Work out the finished part from the listing and answer in its coordinate system (mm). A direction names the side the tool comes from. Give positions to 0.01 mm unless a question says otherwise; leave off trailing zeros. Order: outer loops, then holes, each group sorted by start corner. A loop starts at its lowest first (then second) coordinate and runs counter-clockwise, first axis right, second up. Notation, with made-up numbers: (-4, 7.5) -> (43, 7.5) arc R28 ccw to (43, 36.5) -> close; hole circle Ø1 at (-23, 37). An arc over 180 degrees is marked (long way). Use a Markdown table: item, result. Add a question column.
```python
from build123d import *

# Parameters (mm, degrees)
F0_W     = 32.913417
F0_H     = 15.983271
F0_R     = 0.5
F0_R_2   = 1
F0_R_3   = 1.5
F0_R_4   = 2
F0_R_5   = 2.5
F1_DEPTH = 2
F2_R     = 0.5
F2_R_2   = 1
F2_R_3   = 1.5
F2_R_4   = 2
F2_R_5   = 2.5
F3_DEPTH = 2


with BuildPart() as f1:
    # F0 (on Top) → F1 (new body)
    with BuildSketch(Plane.XY):
        with Locations((16.456708, 7.991635)):
            Rectangle(F0_W, F0_H)
        with Locations((3.5, 3.5)):
            Circle(F0_R, mode=Mode.SUBTRACT)
        with Locations((7.972136, 4)):
            Circle(F0_R_2, mode=Mode.SUBTRACT)
        with Locations((13.449362, 4.5)):
            Circle(F0_R_3, mode=Mode.SUBTRACT)
        with Locations((19.930102, 5)):
            Circle(F0_R_4, mode=Mode.SUBTRACT)
        with Locations((27.413417, 5.5)):
            Circle(F0_R_5, mode=Mode.SUBTRACT)
        with Locations((5.5, 10.483271)):
            Circle(F0_R_5, mode=Mode.SUBTRACT)
        with Locations((12.983315, 10.983271)):
            Circle(F0_R_4, mode=Mode.SUBTRACT)
        with Locations((19.464055, 11.483271)):
            Circle(F0_R_3, mode=Mode.SUBTRACT)
        with Locations((24.941281, 11.983271)):
            Circle(F0_R_2, mode=Mode.SUBTRACT)
        with Locations((29.413417, 12.483271)):
            Circle(F0_R, mode=Mode.SUBTRACT)
        with Locations((5.5, 10.483271)):
            Circle(F0_R_5)
        with Locations((12.983315, 10.983271)):
            Circle(F0_R_4)
        with Locations((19.464055, 11.483271)):
            Circle(F0_R_3)
        with Locations((24.941281, 11.983271)):
            Circle(F0_R_2)
        with Locations((29.413417, 12.483271)):
            Circle(F0_R)
    extrude(amount=F1_DEPTH)

    # F2 (on face) → F3 (join)
    with BuildSketch(Plane.XY.offset(2)):
        with Locations((29.413417, 12.483271)):
            Circle(F2_R)
        with Locations((24.941281, 11.983271)):
            Circle(F2_R_2)
        with Locations((19.464055, 11.483271)):
            Circle(F2_R_3)
        with Locations((12.983315, 10.983271)):
            Circle(F2_R_4)
        with Locations((5.5, 10.483271)):
            Circle(F2_R_5)
    extrude(amount=F3_DEPTH)


solid = f1.part
```
1) Flat-ended cylindrical pins translate along their axes: pin 1 (5 mm diameter, centred on x = 28, y = 4, fed in from +Z); pin 2 (4.5 mm diameter, centred on x = 27.41, y = 5.5, fed in from +Z); pin 3 (1 mm diameter, centred on y = 12, z = 3.5, fed in from -X). Find the tip coordinate at first contact, or state that the pin passes through.
2) The part is cut by section B-B, the plane x = 8.5. Determine the outline of the cut face in (y, z), then the cut area to 3 significant figures.
3) The part is cut by section A-A, the plane y = 7.5. Determine the outline of the cut face in (x, z).
4) Which of the six approach directions +Z, -Z, +X, -X, +Y, -Y give full straight-line access (tool end or side, diameter ignored) to faces 5 (the cylindrical face through (17.966, 11.549, 2.986)), 6 (the cylindrical face through (14.835, 3.925, 0.986))?
5) Straight lines are drawn through the part: line 1 (Z direction, x = 29.5, y = 10.5); line 2 (Y direction, x = 28.5, z = 1.5); line 3 (Y direction, x = 19.5, z = 3.35). For each, find the intervals that lie inside material, in ascending order.
6) The part is cut by section C-C, the plane z = 1.1. Determine the outline of the cut face in (x, y).
7) The part is cut by section D-D, the plane y = 4.5. Determine the outline of the cut face in (x, z).
8) Determine the mould class of faces 1 (the flat face through (0, 8, 1)), 2 (the cylindrical face through (14.891, 11.584, 2.986)), 3 (the flat face through (32.913, 8, 1)), 4 (the flat face through (13, 11, 4)) for opening direction X: released by +X, released by -X, zero draft, split by the parting line, or undercut.
A:
| question | item | result |
|---|---|---|
| 1 | pin 1 | z = 2 |
| 1 | pin 2 | through |
| 1 | pin 3 | x = 3.22 |
| 2 | outline | (0, 0) -> (3.15, 0) -> (3.15, 2) -> (0, 2) -> close; (4.85, 0) -> (15.98, 0) -> (15.98, 2) -> (4.85, 2) -> close |
| 2 | area | 28.6 mm^2 |
| 3 | outline | (0, 0) -> (25.91, 0) -> (25.91, 2) -> (0, 2) -> close; (28.91, 0) -> (32.91, 0) -> (32.91, 2) -> (28.91, 2) -> close |
| 4 | face 5 | +Z |
| 4 | face 6 | +Z, -Z |
| 5 | line 1 | 0 to 2 |
| 5 | line 2 | 0 to 3.25, 7.75 to 15.98 |
| 5 | line 3 | 9.98 to 12.98 |
| 6 | outline | (0, 0) -> (32.91, 0) -> (32.91, 15.98) -> (0, 15.98) -> close; hole circle Ø1 at (3.5, 3.5); hole circle Ø2 at (7.97, 4); hole circle Ø3 at (13.45, 4.5); hole circle Ø4 at (19.93, 5); hole circle Ø5 at (27.41, 5.5) |
| 7 | outline | (0, 0) -> (7.11, 0) -> (7.11, 2) -> (0, 2) -> close; (8.84, 0) -> (11.95, 0) -> (11.95, 2) -> (8.84, 2) -> close; (14.95, 0) -> (17.99, 0) -> (17.99, 2) -> (14.95, 2) -> close; (21.87, 0) -> (25.12, 0) -> (25.12, 2) -> (21.87, 2) -> close; (29.7, 0) -> (32.91, 0) -> (32.91, 2) -> (29.7, 2) -> close |
| 8 | face 1 | released by -X |
| 8 | face 2 | undercut |
| 8 | face 3 | released by +X |
| 8 | face 4 | zero draft |
